Design review of the part shown in the three views and the two pictorial views. Dimensions are in mm from the part's minimum x, y and z. A direction names the side the tool comes from. Coordinates: 2 decimals unless noted, no trailing zeros. Order: outer loops, then holes, each group sorted by start corner. A loop starts at its lowest first (then second) coordinate and runs counter-clockwise, first axis right, second up. Notation, with made-up numbers: (-32, 14) -> (-15, 14) arc R15 ccw to (-15, 42) -> close; hole circle Ø5 at (71, -6.75). An arc over 180 degrees is marked (long way). Answer as a JSON object with one key per item and string values. Group by question number.
1) Add section B-B, the plane x = 3.8. Write out the cut boundary in (y, z).
2) Add section A-A, the plane z = 31. Write out the cut boundary in (x, y), then the cut area to 3 significant figures.
3) Add section C-C, the plane y = 56. Write out the cut boundary in (x, z).
4) Add section D-D, the plane y = 63. Write out the cut boundary in (x, z).
5) Machinability: for the marked faces 1, 2 and 3, which of the approach directions +Z, -Z, +X, -X, +Y, -Y give a long, thin tool a straight path to every point of the face, cutting with its end or side? Answer none if there is none.
6) For pin 1 (1.5 mm diameter, centred on x = 2.5, z = 28.5, fed in from +Y); pin 2 (2.5 mm diameter, centred on y = 60, z = 10, fed in from -X); pin 3 (3 mm diameter, centred on x = 3, z = 16, fed in from +Y), all flat-tipped, find the tip position at first contact; note any pin that passes through.
7) Wall thickness on L1, parallel to Y at x = 1.6, z = 10; L2, parallel to Y at x = 1.75, z = 30.5; L3, parallel to Y at x = 2.55, z = 20.5: over which ranges is each line inside the solid? List them lowest first.
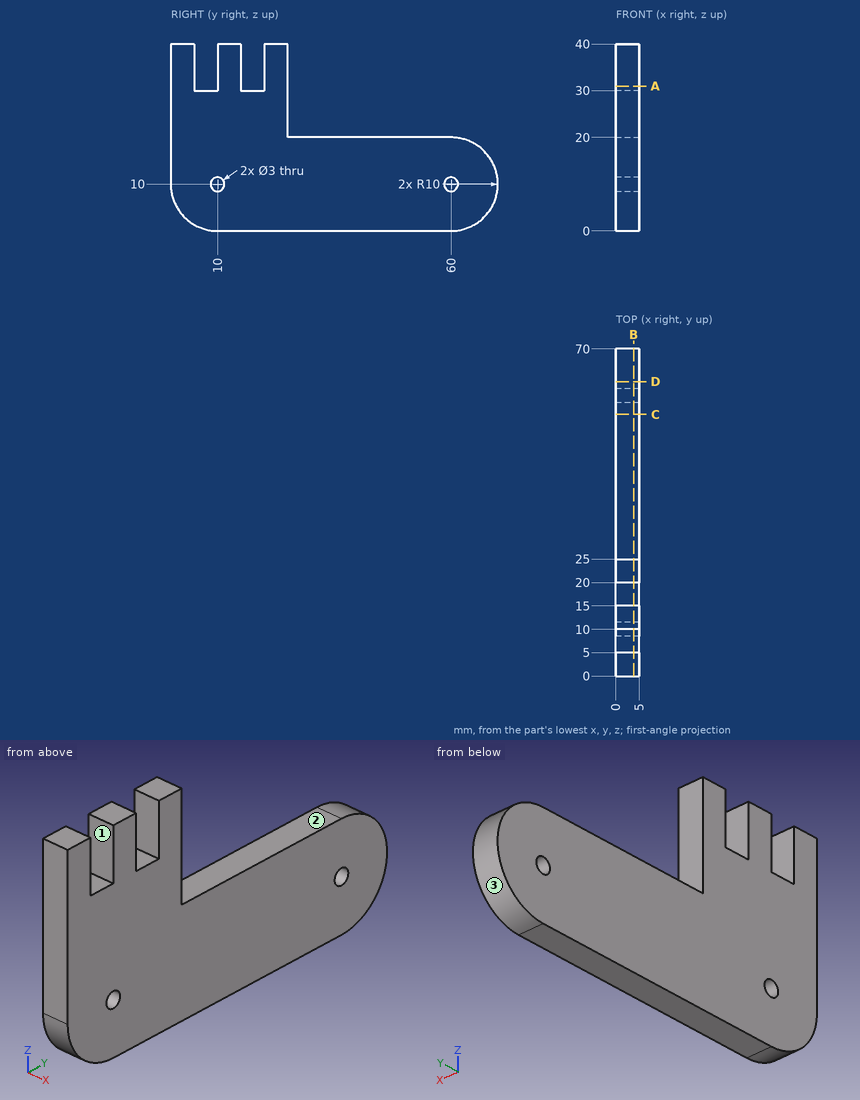
Output values:
{
 "1": {"outline": "(0, 10) arc R10 ccw to (10, 0) -> (60, 0) arc R10 ccw to (60, 20) -> (25, 20) -> (25, 40) -> (20, 40) -> (20, 30) -> (15, 30) -> (15, 40) -> (10, 40) -> (10, 30) -> (5, 30) -> (5, 40) -> (0, 40) -> close; hole circle Ø3 at (10, 10); hole circle Ø3 at (60, 10)"},
 "2": {"outline": "(0, 0) -> (5, 0) -> (5, 5) -> (0, 5) -> close; (0, 10) -> (5, 10) -> (5, 15) -> (0, 15) -> close; (0, 20) -> (5, 20) -> (5, 25) -> (0, 25) -> close", "area": "75.0 mm²"},
 "3": {"outline": "(0, 0) -> (5, 0) -> (5, 20) -> (0, 20) -> close"},
 "4": {"outline": "(0, 0.46) -> (5, 0.46) -> (5, 19.54) -> (0, 19.54) -> close"},
 "5": {"face 1": "+Z, +X, -X", "face 2": "+Z, +X, -X, +Y", "face 3": "+X, -X, +Y"},
 "6": {"pin 1": "stops at y = 25", "pin 2": "passes through", "pin 3": "stops at y = 68.93"},
 "7": {"L1": "y = 0 to 8.5, 11.5 to 58.5, 61.5 to 70", "L2": "y = 0 to 5, 10 to 15, 20 to 25", "L3": "y = 0 to 25"}
}
